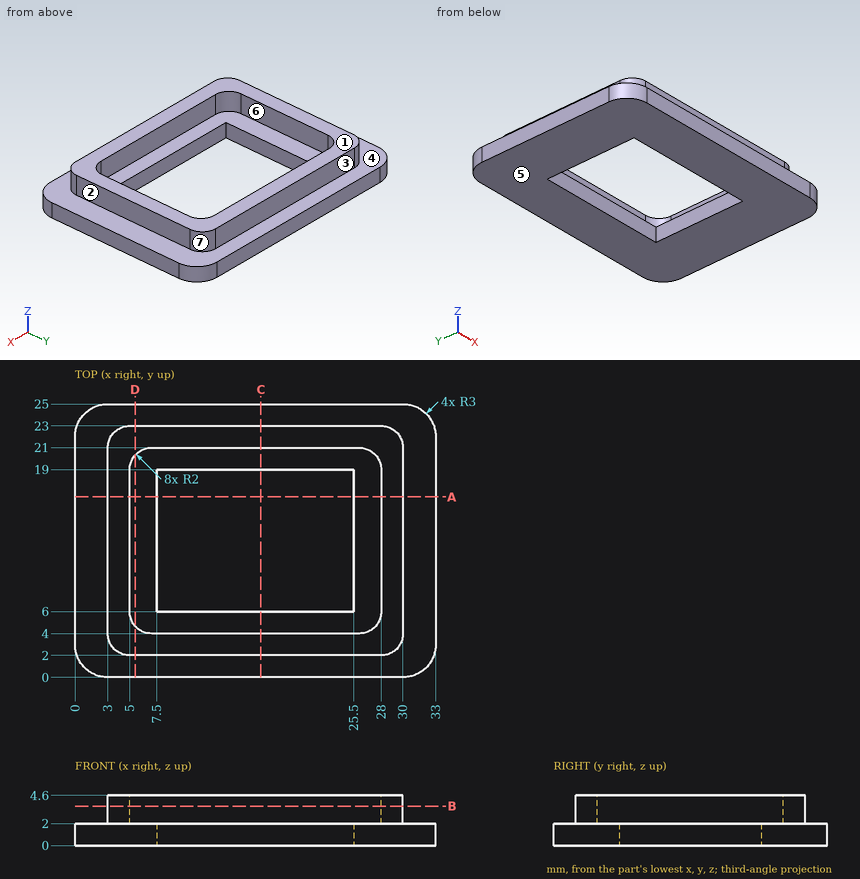
Geometry: see drawing. Coordinates: mm, zero at the bounding-box minimum. A direction names the side the tool comes from. Round coordinates to 2 decimals unless told otherwise and drop trailing zeros. Loops run counter-clockwise (first coordinate to the right, second up) from the corner with the lowest first, then second, coordinate; pieces in that order, holes last. Notation, with made-up numbers: (-29.75, 9) -> (17.25, 9) arc R33 cw to (17.25, 48) -> close; hole circle Ø4 at (42.5, 68). An arc over 180 degrees is marked (long way). Use one line per item in the form item = value. Start each with the question number.
Item 1: Mould query, pull axis X, two halves, no side actions, for the marked faces 5, 6 and 7. Classes: pulls with the +X half, pulls with the -X half, needs draft (parallel to the pull), parting line crosses it, or undercut.
Item 2: Section query B-B on z = 3.6. Return the cut outline in (x, y), then the cut area to 3 significant figures.
Item 3: Set-up query: the marked faces 1, 2, 3 and 4. Return all of +Z, -Z, +X, -X, +Y, -Y with unobstructed straight access to the full face (end or side cutting, diameter ignored); none if empty.
Item 4: Section query D-D on x = 5.5. Return the cut outline in (y, z).
Item 5: Section query A-A on y = 16.5. Return the cut outline in (x, z).
Item 6: Section query C-C on x = 17. Return the cut outline in (y, z).
Item 7: Contact query for flat-ended pins moving along their axis: pin 1 Ø1.3 at (y, z) = (9.5, 3.5) entering from -X; pin 2 Ø0.8 at (x, z) = (22, 2.5) entering from -Y; pin 3 Ø0.8 at (x, z) = (12.5, 3) entering from +Y. Output: stop coordinate, or through.
Item 8: Material intervals for L1, parallel to X at y = 12.5, z = 1.4; L2, parallel to Y at x = 26, z = 3.3; L3, parallel to X at y = 18.5, z = 2.25, sorted ascending. Write a range as from..to.
Ans:
q1.face_5 = needs draft
q1.face_6 = undercut
q1.face_7 = pulls with the +X half
q2.outline = (3, 4) arc R2 ccw to (5, 2) -> (28, 2) arc R2 ccw to (30, 4) -> (30, 21) arc R2 ccw to (28, 23) -> (5, 23) arc R2 ccw to (3, 21) -> close; hole (5, 6) arc R2 ccw to (7, 4) -> (26, 4) arc R2 ccw to (28, 6) -> (28, 19) arc R2 ccw to (26, 21) -> (7, 21) arc R2 ccw to (5, 19) -> close
q2.area = 176 mm^2
q3.face_1 = +Z, +X, -X, +Y, -Y
q3.face_2 = +Z, +X, +Y, -Y
q3.face_3 = +Z, +X, -X, +Y
q3.face_4 = +Z
q4.outline = (0, 0) -> (25, 0) -> (25, 2) -> (23, 2) -> (23, 4.6) -> (20.32, 4.6) -> (20.32, 2) -> (4.68, 2) -> (4.68, 4.6) -> (2, 4.6) -> (2, 2) -> (0, 2) -> close
q5.outline = (0, 0) -> (7.5, 0) -> (7.5, 2) -> (5, 2) -> (5, 4.6) -> (3, 4.6) -> (3, 2) -> (0, 2) -> close; (25.5, 0) -> (33, 0) -> (33, 2) -> (30, 2) -> (30, 4.6) -> (28, 4.6) -> (28, 2) -> (25.5, 2) -> close
q6.outline = (0, 0) -> (6, 0) -> (6, 2) -> (4, 2) -> (4, 4.6) -> (2, 4.6) -> (2, 2) -> (0, 2) -> close; (19, 0) -> (25, 0) -> (25, 2) -> (23, 2) -> (23, 4.6) -> (21, 4.6) -> (21, 2) -> (19, 2) -> close
q7.pin_1 = 3
q7.pin_2 = 2
q7.pin_3 = 23
q8.L1 = 0..7.5, 25.5..33
q8.L2 = 2..4, 21..23
q8.L3 = 3..5, 28..30
